CAD build for the part. Positions are in the model's coordinates, mm. A direction names the side the tool comes from. Give positions to 0.01 mm unless a question says otherwise; leave off trailing zeros. Loops run counter-clockwise (first coordinate to the right, second up) from the corner with the lowest first, then second, coordinate; pieces in that order, holes last. Notation, with made-up numbers: M -1.75,-18 L 50.25,-18 A12 ccw 50.25,-6 Z; hole C 45.25,57 d1. An arc over 180 degrees is marked long. Answer as CSV lines item,"result".
Autodesk Inventor part; units mm, degrees
ref_plane "YZ Plane" through (0, 0, 0) normal (1, 0, 0) x (0, 1, 0)
ref_plane "XZ Plane" through (0, 0, 0) normal (0, 1, 0) x (-1, 0, 0)
ref_plane "XY Plane" through (0, 0, 0) normal (0, 0, 1) x (1, 0, 0)
ref_plane "Work Plane5" through (0, 0, 10) normal (0, 0, 1) x (1, 0, 0)
sketch "Sketch1" plane through (0, 0, 10) normal (0, 0, 1) x (1, 0, 0)
  line L0 (-4.0299, -0.3538) -> (-2.2322, 1.4439) construction
  arc A0 (-1.4439, 2.2322) -> (-2.2322, 1.4439) centre (-0.9299, 0.9299) ccw construction
  line L1 (-1.4439, 2.2322) -> (0.3538, 4.0299) construction
  line L2 (-37.8299, 42.8299) -> (-37.8299, 37.8299) construction
  line L3 (-37.8299, 37.8299) -> (-42.9208, 37.8299) construction
  line L4 (-37.8299, 42.2137) -> (-37.8299, 45.8299) construction
  line L5 (-37.8299, 45.8299) -> (-4.0299, 45.8299) construction
  line L6 (-4.0299, 45.8299) -> (-4.0299, 42.2137) construction
  line L7 (-4.0299, 4.0299) -> (0.3538, 4.0299)
  circle A1 centre (-20.9299, 20.9299) radius 17.5
  line L8 (-20.9299, 58.9723) -> (17.1124, 20.9299) construction
  line L9 (17.1124, 20.9299) -> (-20.9299, -17.1124) construction
  line L10 (-20.9299, -17.1124) -> (-58.9723, 20.9299) construction
  line L11 (-58.9723, 20.9299) -> (-20.9299, 58.9723) construction
  line L12 (-20.9299, 58.9723) -> (-20.9299, -17.1124) construction
  line L13 (17.1124, 20.9299) -> (-58.9723, 20.9299) construction
  line L14 (-20.9299, 58.9723) -> (32.8701, 58.9723) construction
  line L15 (-43.4299, 43.4299) -> (1.5701, 43.4299) construction
  line L16 (1.5701, 43.4299) -> (1.5701, -1.5701) construction
  line L17 (1.5701, -1.5701) -> (-43.4299, -1.5701) construction
  line L18 (-43.4299, -1.5701) -> (-43.4299, 43.4299) construction
  line L19 (-43.4299, 43.4299) -> (1.5701, -1.5701) construction
  line L20 (1.5701, 43.4299) -> (-43.4299, -1.5701) construction
  line L21 (-43.4299, 5.3876) -> (-43.4299, 36.4723)
  line L22 (-43.4299, 36.4723) -> (-36.4723, 43.4299)
  line L23 (-36.4723, 43.4299) -> (-5.3876, 43.4299)
  line L24 (-5.3876, 43.4299) -> (1.5701, 36.4723)
  line L25 (1.5701, 36.4723) -> (1.5701, 5.3876)
  line L26 (1.5701, 5.3876) -> (-5.3876, -1.5701)
  line L27 (-5.3876, -1.5701) -> (-36.4723, -1.5701)
  line L28 (-36.4723, -1.5701) -> (-43.4299, 5.3876)
  line L29 (-4.0299, 42.2137) -> (-37.8299, 42.2137)
  line L30 (-4.0299, -0.3538) -> (-4.0299, 4.0299)
  circle A2 centre (-20.9299, 20.9299) radius 1.5
  line L31 (-10.9299, 10.9299) -> (-30.9299, 10.9299) construction
  line L32 (-30.9299, 10.9299) -> (-30.9299, 30.9299) construction
  line L33 (-30.9299, 30.9299) -> (-10.9299, 30.9299) construction
  line L34 (-10.9299, 30.9299) -> (-10.9299, 10.9299) construction
  line L35 (-10.9299, 10.9299) -> (-30.9299, 30.9299) construction
  line L36 (-30.9299, 10.9299) -> (-10.9299, 30.9299) construction
  circle A3 centre (-30.9299, 30.9299) radius 1.4
  circle A4 centre (-30.9299, 10.9299) radius 1.4
  circle A5 centre (-10.9299, 10.9299) radius 1.4
  line L37 (-45.8299, 37.8299) -> (-42.0723, 37.8299) construction
  line L38 (-42.1723, 37.7299) -> (-45.8299, 37.7299)
  line L39 (-45.8299, 37.7299) -> (-45.8299, 4.1299)
  line L40 (-45.8299, 4.1299) -> (-42.1723, 4.1299)
  line L41 (-42.1723, 4.1299) -> (-42.1723, 37.7299)
  line L42 (-45.8299, 4.0299) -> (-42.0723, 4.0299) construction
  line L43 (-45.8299, 37.8299) -> (-42.0723, 37.8299)
  line L44 (-37.7299, 45.8299) -> (-4.1299, 45.8299)
  line L45 (-4.1299, 45.8299) -> (-4.1299, 42.1723)
  line L46 (-4.1299, 42.1723) -> (-37.7299, 42.1723)
  line L47 (-37.7299, 42.1723) -> (-37.7299, 45.8299)
  line L48 (0.4701, 37.8299) -> (0.4701, 4.0299) construction
  line L49 (0.4701, 4.0299) -> (3.9701, 4.0299) construction
  line L50 (3.9701, 37.8299) -> (3.9701, 4.0299) construction
  line L51 (0.4701, 37.8299) -> (3.9701, 37.8299) construction
  line L52 (-45.8299, -3.9701) -> (-4.0299, -3.9701) construction
  line L53 (0.3124, 37.7299) -> (3.9701, 37.7299)
  line L54 (3.9701, 37.7299) -> (3.9701, 4.1299)
  line L55 (3.9701, 4.1299) -> (0.3124, 4.1299)
  line L56 (0.3124, 4.1299) -> (0.3124, 37.7299)
  line L57 (-4.1713, -0.3538) -> (-37.7299, -0.3538)
  line L58 (-37.7299, -0.3538) -> (-37.7299, -3.9701)
  line L59 (-37.7299, -3.9701) -> (-4.1713, -3.9701)
  line L60 (-4.1713, -3.9701) -> (-4.1713, -0.3538)
  point P0 (-37.8299, 4.0299)
  dimension "d18" = 53.8
  dimension "d19" = 45
  dimension "d20" = 53.8
  dimension "d21" = 45
  dimension "d22" = 45
  dimension "d30" = 20
  dimension "d31" = 20
  dimension "d32" = 2.8
  dimension "d33" = 2.8
  dimension "d34" = 2.8
  dimension "d35" = 3
  dimension "d36" = 0.1
  dimension "d37" = 0.1
  dimension "d38" = 0.1
  dimension "d39" = 0.1
extrude "Extrusion1" add sketch "Sketch1" along normal blind 15 contours L30 L26 L57 L28 L41 L22 L46 L24 L56 L7 | L7 L26 L30 | L56 L24 L25 L26 | L26 L25 L24 L53 L54 L55 | L60 L59 L58 L57 L28 L27 L26 | L26 L27 L28 L57 | L46 L22 L29 L24 | L24 L29 L45 | L40 L39 L38 L22 L21 L28 | L28 L21 L22 L41 | L29 L22 L23 L24 | L24 L23 L22 L29 L47 L44 L45 | L47 L29 L22 | A1 | A2 | A3 | A4 | A5
sketch "Skizze4" plane through (0, 0, 25) normal (0, 0, 1) x (1, 0, 0)
  line L0 (-37.7299, 42.1723) -> (-42.1723, 37.7299)
  line L1 (-42.1723, 37.7299) -> (-45.8299, 37.7299)
  line L2 (-45.8299, 37.7299) -> (-45.8299, 4.1299) construction
  line L3 (-45.8299, 4.1299) -> (-42.1723, 4.1299)
  line L4 (-42.1723, 4.1299) -> (-37.6885, -0.3538)
  line L5 (-37.6885, -0.3538) -> (-37.7299, -0.3538)
  line L6 (-37.7299, -0.3538) -> (-37.7299, -3.9701)
  line L7 (-37.7299, -3.9701) -> (-4.1713, -3.9701) construction
  line L8 (-4.1713, -3.9701) -> (-4.1713, -0.3538)
  line L9 (-4.1713, -0.3538) -> (0.3124, 4.1299)
  line L10 (0.3124, 4.1299) -> (3.9701, 4.1299)
  line L11 (3.9701, 4.1299) -> (3.9701, 37.7299) construction
  line L12 (3.9701, 37.7299) -> (0.3124, 37.7299)
  line L13 (0.3124, 37.7299) -> (-4.1299, 42.1723)
  line L14 (-4.1299, 42.1723) -> (-4.1299, 45.8299)
  line L15 (-4.1299, 45.8299) -> (-37.7299, 45.8299) construction
  line L16 (-37.7299, 45.8299) -> (-37.7299, 42.1723)
  line L17 (-37.9299, 46.0299) -> (-3.9299, 46.0299) construction
  line L18 (-3.9299, 46.0299) -> (-3.9299, 42.2551)
  line L19 (-3.9299, 42.2551) -> (0.3953, 37.9299)
  line L20 (0.3953, 37.9299) -> (4.1701, 37.9299)
  line L21 (4.1701, 37.9299) -> (4.1701, 3.9299) construction
  line L22 (4.1701, 3.9299) -> (0.3953, 3.9299)
  line L23 (0.3953, 3.9299) -> (-3.9713, -0.4367)
  line L24 (-3.9713, -0.4367) -> (-3.9713, -4.1701)
  line L25 (-3.9713, -4.1701) -> (-37.9299, -4.1701) construction
  line L26 (-37.9299, -4.1701) -> (-37.9299, -0.3953)
  line L27 (-37.9299, -0.3953) -> (-42.2551, 3.9299)
  line L28 (-42.2551, 3.9299) -> (-46.0299, 3.9299)
  line L29 (-46.0299, 3.9299) -> (-46.0299, 37.9299) construction
  line L30 (-46.0299, 37.9299) -> (-42.2551, 37.9299)
  line L31 (-42.2551, 37.9299) -> (-37.9299, 42.2551)
  line L32 (-37.9299, 42.2551) -> (-37.9299, 46.0299)
  line L33 (-45.8299, 37.7299) -> (-45.8299, 37.9299)
  line L34 (-4.1299, 45.8299) -> (-37.7299, 45.8299)
  line L35 (-37.7299, 45.8299) -> (-37.9299, 45.8299)
  line L36 (-4.1299, 45.8299) -> (-3.9299, 45.8299)
  line L37 (3.9701, 37.7299) -> (3.9701, 37.9299)
  line L38 (3.9701, 4.1299) -> (3.9701, 37.7299)
  line L39 (3.9701, 4.1299) -> (3.9701, 3.9299)
  line L40 (-4.1713, -3.9701) -> (-3.9713, -3.9701)
  line L41 (-37.7299, -3.9701) -> (-37.9299, -3.9701)
  line L42 (-45.8299, 4.1299) -> (-45.8299, 3.9299)
  point P0 (0, 0)
  dimension "d40" = 0.2
extrude "IM_offset" add sketch "Skizze4" against normal up to surface (15 mm away)
sketch "Sketch29" plane through (0, 0, 10) normal (0, 0, -1) x (-1, 0, 0)
  line L0 (9.4299, 6.9299) -> (32.4299, 6.9299)
  arc A0 (6.9299, 9.4299) -> (9.4299, 6.9299) centre (9.4299, 9.4299) ccw
  line L1 (6.9299, 32.4299) -> (6.9299, 9.4299)
  arc A1 (9.4299, 34.9299) -> (6.9299, 32.4299) centre (9.4299, 32.4299) ccw
  line L2 (32.4299, 34.9299) -> (9.4299, 34.9299)
  arc A2 (34.9299, 32.4299) -> (32.4299, 34.9299) centre (32.4299, 32.4299) ccw
  line L3 (34.9299, 9.4299) -> (34.9299, 32.4299)
  arc A3 (32.4299, 6.9299) -> (34.9299, 9.4299) centre (32.4299, 9.4299) ccw
  circle A4 centre (20.9299, 20.9299) radius 11
  circle A5 centre (9.4299, 32.4299) radius 1.025
  circle A6 centre (9.4299, 9.4299) radius 1.025
  circle A7 centre (32.4299, 9.4299) radius 1.025
  circle A8 centre (32.4299, 32.4299) radius 1.025
  arc A9 (6.7299, 9.4299) -> (9.4299, 6.7299) centre (9.4299, 9.4299) ccw
  line L4 (9.4299, 6.7299) -> (32.4299, 6.7299)
  arc A10 (32.4299, 6.7299) -> (35.1299, 9.4299) centre (32.4299, 9.4299) ccw
  line L5 (35.1299, 9.4299) -> (35.1299, 32.4299)
  arc A11 (35.1299, 32.4299) -> (32.4299, 35.1299) centre (32.4299, 32.4299) ccw
  line L6 (32.4299, 35.1299) -> (9.4299, 35.1299)
  arc A12 (9.4299, 35.1299) -> (6.7299, 32.4299) centre (9.4299, 32.4299) ccw
  line L7 (6.7299, 32.4299) -> (6.7299, 9.4299)
  point P0 (0, 0)
  dimension "d176" = 0.2
extrude "Extrusion23" cut sketch "Sketch29" against normal through all contours A0 L1 A1 L2 A2 L3 A3 L0 | A4 | A5 | A6 | A7 | A8 | L7 A12 L6 A11 L5 A10 L4 A9
sketch "Sketch30" plane through (-45.8299, 0, 10) normal (-1, 0, 0) x (0, 0, 1)
  line L0 (35.0799, 45.8299) -> (6.8799, 45.8299)
  line L1 (0, 3.9299) -> (0, 37.9299)
  line L2 (15, 3.9299) -> (0, 3.9299)
  line L3 (15, 37.9299) -> (15, 3.9299)
  line L4 (15, 37.9299) -> (0, 37.9299)
  circle A0 centre (5, 20.9299) radius 1.7201
  point P0 (-10, 0)
ref_plane "Arbeitsebene7" through (-20.9299, 3.9299, 10) normal (-1, 0, 0) x (0, 0, 1)
ref_plane "Arbeitsebene8" through (-37.9299, 20.9299, 10) normal (0, 1, 0) x (1, 0, 0)
ref_plane "Arbeitsebene9" through (-20.9299, 3.9299, 10) normal (-1, 0, 0) x (0, 0, 1)
ref_plane "Arbeitsebene10" through (-37.9299, 20.9299, 10) normal (0, -1, 0) x (1, 0, 0)
hole "Bohrung2" at (-45.8299, 20.9299, 15) direction (1, 0, 0) diameter 2.8 end through all counterbore diameter 6 counterbore depth 4
pattern_circular "Runde Anordnung2" count 4 over 360 about axis through (-20.9299, 20.9299, 10) along (0, 0, 1) of "Bohrung2"
ref_plane "Arbeitsebene11" through (-20.9299, 3.9299, 10) normal (1, 0, 0) x (0, 0, -1)
ref_plane "Arbeitsebene12" through (-37.9299, 20.9299, 10) normal (0, 1, 0) x (1, 0, 0)
properties part number "30_Cube_Z_Focus_MGN_NEMA_Motorsupport_centered"
1) Mould opens along Y. For faces 4 (the face through (-21, 6.73, 17)), 5 (the face through (-7.5, 7.54, 17.4)), 6 (the face through (-21.6, 0.03, 13.6)), 7 (the face through (3.97, 21, 19)) say: +Y half, -Y half, draft (parallel to the pull), parting line (faces both ways), or undercut.
Answer below:
face 4,"undercut"
face 5,"undercut"
face 6,"-Y half"
face 7,"draft"
2) Band-saw the part on B-B on z = 15. Give the number of separate pieces and of enclosed holes in the cut face, and give its area (3 significant figures).
Answer below:
separate pieces,"4"
enclosed holes,"0"
area,"1,300 mm^2"
3) Band-saw the part on A-A on y = 13.5. Give the cut face in (x, z).
Answer below:
outline,"M -45.83,10 L -35.13,10 L -35.13,25 L -45.83,25 Z; M -6.73,10 L 3.97,10 L 3.97,25 L -6.73,25 Z"
4) Band-saw the part on C-C on y = 8. Give the cut face in (x, z), and give its area (3 significant figures).
Answer below:
outline,"M -45.83,10 L -34.72,10 L -34.72,25 L -45.83,25 Z; M -7.14,10 L 3.97,10 L 3.97,25 L -7.14,25 Z"
area,"333 mm^2"
5) Flat gauge pins, fed straight in: pin 1 (3.5 mm diameter, centred on y = 20.93, z = 15, fed in from -X); pin 2 (3 mm diameter, centred on x = 2.5, z = 14.5, fed in from -Y); pin 3 (4 mm diameter, centred on x = -18.5, z = 16, fed in from -Y); pin 4 (2.5 mm diameter, centred on x = -20.93, z = 15, fed in from +Y). Where does each tip first touch, or does it go through?
Answer below:
pin 1,"stops at x = -41.83"
pin 2,"stops at y = 3.93"
pin 3,"stops at y = -3.97"
pin 4,"passes through"
6) Which spindle directions (+Z, -Z, +X, -X, +Y, -Y) get a long thin tool onto all of the face, cutting with end or side? Do faces 1 (the face through (-44, 37.93, 18)), 2 (the face through (-7.54, 34.36, 17.4)), 3 (the face through (-37.93, -2, 18)). Say none if no direction does.
Answer below:
face 1,"+Z, -Z, -X, +Y"
face 2,"+Z, -Z"
face 3,"+Z, -Z, -X, -Y"
7) Drill centre lines: line 1 (X direction, y = 32, z = 22.5); line 2 (Y direction, x = -23, z = 24.25); line 3 (X direction, y = 33.5, z = 19). Where is each one in solid material? Low to high. Write a range as from..to.
Answer below:
line 1,"x = -45.83..-35.13, -6.73..3.97"
line 2,"y = -3.97..6.73, 35.13..45.83"
line 3,"x = -45.83..-34.91, -6.95..3.97"
